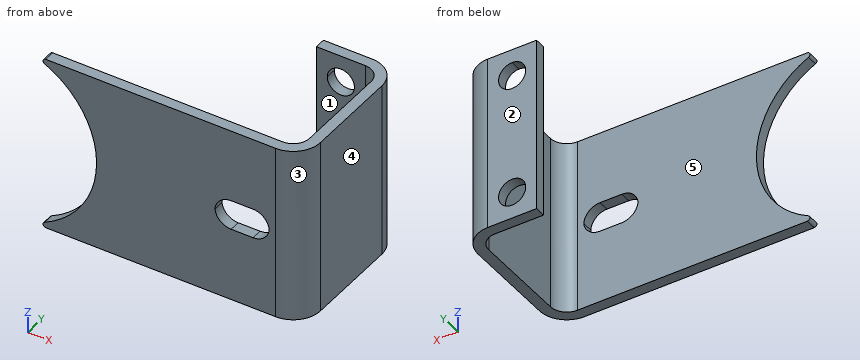
from build123d import *

# Parameters (mm, degrees)
F1_DEPTH = 65
F3_DEPTH = 25
F5_DEPTH = 25
F6_DEPTH = 11
F7_R     = 1
F8_R     = 1


with BuildPart() as f1:
    # F0 (on Top) → F1 (new body)
    with BuildSketch(Plane.XY):
        with BuildLine():
            Line((28.8081228733, 30.691023916), (10.8081228733, 30.691023916))
            Line((10.8081228733, 30.691023916), (10.8081228733, 26.691023916))
            Line((10.8081228733, 26.691023916), (28.8081228733, 26.691023916))
            ThreePointArc((28.8081228733, 26.691023916), (33.0507635604, 24.9336646031), (34.8081228733, 20.691023916))
            Line((34.8081228733, 20.691023916), (34.8081228733, 19.2851312459))
            Line((34.8081228733, 19.2851312459), (34.8081228733, -14.308976084))
            ThreePointArc((34.8081228733, -14.308976084), (33.0507635604, -18.5516167711), (28.8081228733, -20.308976084))
            Line((28.8081228733, -20.308976084), (-71.1918771267, -20.308976084))
            Line((-71.1918771267, -20.308976084), (-71.1918771267, -22.308976084))
            Line((-71.1918771267, -22.308976084), (-71.1918771267, -24.308976084))
            Line((-71.1918771267, -24.308976084), (28.8081228733, -24.308976084))
            ThreePointArc((28.8081228733, -24.308976084), (35.8791906852, -21.3800438959), (38.8081228733, -14.308976084))
            Line((38.8081228733, -14.308976084), (38.8081228733, 20.691023916))
            ThreePointArc((38.8081228733, 20.691023916), (35.8791906852, 27.7620917279), (28.8081228733, 30.691023916))
        make_face()
    extrude(amount=F1_DEPTH)

    # F2 (on face) → F3 (cut)
    with BuildSketch(Plane(origin=(0, 30.691023916, 0), x_dir=(-1, 0, 0), z_dir=(0, 1, 0))):
        with BuildLine():
            ThreePointArc((-14.8081228733, 55), (-16.2725889674, 58.5355339059), (-19.8081228733, 60))
            ThreePointArc((-19.8081228733, 60), (-23.3436567792, 51.4644660941), (-14.8081228733, 55))
        make_face()
        with BuildLine():
            ThreePointArc((-14.8081228733, 10), (-23.3436567792, 13.5355339059), (-19.8081228733, 5))
            ThreePointArc((-19.8081228733, 5), (-16.2725889674, 6.4644660941), (-14.8081228733, 10))
        make_face()
    extrude(amount=-F3_DEPTH, mode=Mode.SUBTRACT)

    # F4 (on face) → F5 (cut)
    with BuildSketch(Plane(origin=(0, -20.308976084, 0), x_dir=(-1, 0, 0), z_dir=(0, 1, 0))):
        with BuildLine():
            ThreePointArc((-6.4388471842, 32.5), (-8.3123065892, 36.4995007653), (-12.4155679156, 38.1332397291))
            Line((-12.4155679156, 38.1332397291), (-20.4500670994, 38.1332397291))
            ThreePointArc((-20.4500670994, 38.1332397291), (-24.5609939033, 36.5036265326), (-26.4388471842, 32.5))
            ThreePointArc((-26.4388471842, 32.5), (-24.4848723268, 28.6723295991), (-20.4723568049, 27.1332397291))
            Line((-20.4723568049, 27.1332397291), (-12.4053375634, 27.1332397291))
            ThreePointArc((-12.4053375634, 27.1332397291), (-8.3928220416, 28.6723295991), (-6.4388471842, 32.5))
        make_face()
    extrude(amount=-F5_DEPTH, mode=Mode.SUBTRACT)

    # F4 (on face) → F6 (cut)
    with BuildSketch(Plane(origin=(0, -20.308976084, 0), x_dir=(-1, 0, 0), z_dir=(0, 1, 0))):
        with BuildLine():
            ThreePointArc((61.204384949, 0), (91.3961497684, 5.1542989298), (105.1918771267, 32.5))
            ThreePointArc((105.1918771267, 32.5), (91.3961497684, 59.8457010702), (61.204384949, 65))
            Line((61.204384949, 65), (71.1918771267, 65))
            Line((71.1918771267, 65), (71.1918771267, 0))
            Line((71.1918771267, 0), (61.204384949, 0))
        make_face()
        with BuildLine():
            Line((71.1918771267, 65), (61.204384949, 65))
            ThreePointArc((61.204384949, 65), (37.1918771267, 32.5), (61.204384949, 0))
            Line((61.204384949, 0), (71.1918771267, 0))
            Line((71.1918771267, 0), (71.1918771267, 65))
        make_face()
    extrude(amount=-F6_DEPTH, mode=Mode.SUBTRACT)

    # F7
    f7_edges = [f1.edges().sort_by_distance(p)[0] for p in [
        (-61.204385, -22.308976, 65),
    ]]
    fillet(f7_edges, radius=F7_R)

    # F8
    f8_edges = [f1.edges().sort_by_distance(p)[0] for p in [
        (-61.204385, -22.308976, 0),
    ]]
    fillet(f8_edges, radius=F8_R)


solid = f1.part
Read the model definition and answer for the solid it produces. Units are mm, in the model's axes. Face numbers are marked on the shaded views. A direction names the side the tool comes from. Coordinates: 2 decimals unless noted, no trailing zeros. Order: outer loops, then holes, each group sorted by start corner. A loop starts at its lowest first (then second) coordinate and runs counter-clockwise, first axis right, second up. Notation, with made-up numbers: M -19.75,-21 L 5.25,-21 A32 ccw 5.25,12 Z; hole C 26.25,-15 d10. An arc over 180 degrees is marked long. Put each result on its own line as item: value. Start each with the question number.
Item 1: For the marked faces 1 and 2, determine the directions among +Z, -Z, +X, -X, +Y, -Y from which every point of the face is accessible in a straight line to the end or side of a thin tool.
Item 2: Consider probe 1 along Y at (x, z) = (27.5, 20); probe 2 along X at (y, z) = (7, 12.5); probe 3 along Y at (x, z) = (17.5, 28). Determine where each line is inside the solid, lowest interval first. Write a range as [from, to].
Item 3: The mould has two halves that part along Y. Classify the marked faces 3, 4 and 5: +Y half, -Y half, draft (parallel to the pull), parting line (faces both ways), or undercut.
Item 4: Section D-D, the plane y = 11 is taken. Determine the outline of the cut face in (x, z), plus the area to 3 significant figures.
Item 5: Section B-B, the plane z = 39.5 is taken. Determine the outline of the cut face in (x, y), plus the area to 3 significant figures.
Item 6: Given pin 1 Ø1 at (x, z) = (9, 52) entering from +Y; pin 2 Ø3 at (y, z) = (27.5, 24) entering from -X, each flat-ended and moving along its own axis, determine where each tip first touches the part or whether it passes through.
Item 7: Section A-A, the plane x = 17 is taken. Determine the outline of the cut face in (y, z), plus the area to 3 significant figures.
Item 8: Section C-C, the plane x = -48.5 is taken. Determine the outline of the cut face in (y, z).
Computed:
1. face 1: +Z, -Z, -X
1. face 2: +Z, -Z, +X, -X, +Y
2. probe 1: y = [-24.31, -20.31], [26.69, 30.69]
2. probe 2: x = [34.81, 38.81]
2. probe 3: y = [26.69, 30.69]
3. face 3: -Y half
3. face 4: draft
3. face 5: undercut
4. outline: M 34.81,0 L 38.81,0 L 38.81,65 L 34.81,65 Z
4. area: 260 mm2
5. outline: M -37.92,-24.31 L 28.81,-24.31 A10 ccw 38.81,-14.31 L 38.81,20.69 A10 ccw 28.81,30.69 L 10.81,30.69 L 10.81,26.69 L 28.81,26.69 A6 cw 34.81,20.69 L 34.81,-14.31 A6 cw 28.81,-20.31 L -37.92,-20.31 Z
5. area: 579 mm2
6. pin 1: stops at y = -20.31
6. pin 2: stops at x = 10.81
7. outline: M -24.31,0 L -20.31,0 L -20.31,27.13 L -24.31,27.13 Z; M -24.31,38.13 L -20.31,38.13 L -20.31,65 L -24.31,65 Z; M 26.69,0 L 30.69,0 L 30.69,5.86 L 26.69,5.86 Z; M 26.69,14.14 L 30.69,14.14 L 30.69,50.86 L 26.69,50.86 Z; M 26.69,59.14 L 30.69,59.14 L 30.69,65 L 26.69,65 Z
7. area: 410 mm2
8. outline: M -24.31,0 L -20.31,0 L -20.31,7.18 L -24.31,7.18 Z; M -24.31,57.82 L -20.31,57.82 L -20.31,65 L -24.31,65 Z
